from build123d import *

# Parameters (mm, degrees)
CYLINDER005_R     = 2
CYLINDER005_DEPTH = 6
CYLINDER004_R     = 52
CYLINDER004_DEPTH = 67
CYLINDER003_R     = 8
CYLINDER003_DEPTH = 5


with BuildPart() as screw_cut:
    # Cylinder005 → Cylinder005 (new body)
    with BuildSketch(Plane(origin=(0, 56, -0.5), x_dir=(1, 0, 0), z_dir=(0, 0, 1))):
        Circle(CYLINDER005_R)
    extrude(amount=CYLINDER005_DEPTH)


with BuildPart() as cylinder:
    # Cylinder004 → Cylinder004 (new body)
    with BuildSketch(Plane.XY):
        Circle(CYLINDER004_R)
    extrude(amount=CYLINDER004_DEPTH)


with BuildPart() as hinge_final:
    # Cylinder003 → Cylinder003 (new body)
    with BuildSketch(Plane(origin=(0, 52, 0), x_dir=(1, 0, 0), z_dir=(0, 0, 1))):
        Circle(CYLINDER003_R)
    extrude(amount=CYLINDER003_DEPTH)

    # Cut002: cut Cylinder
    add(cylinder.part, mode=Mode.SUBTRACT)

    # Cut003: cut Screw Cut
    add(screw_cut.part, mode=Mode.SUBTRACT)


with BuildPart() as part_mirroring:
    # Part__Mirroring: instance of Hinge Final
    add(hinge_final.part.mirror(Plane(origin=(0.001259, 0, 2.5), x_dir=(1, 0, 0), z_dir=(0, 1, 0))))


solid = part_mirroring.part
Source: CAD feature listing. Evaluate the final solid. Frame: model axes, mm. Round coordinates to 2 decimals unless told otherwise and drop trailing zeros. Loops run counter-clockwise (first coordinate to the right, second up) from the corner with the lowest first, then second, coordinate; pieces in that order, holes last. Notation, with made-up numbers: (14.25, 30) - (36.25, 30) arc R6 ccw to (36.25, 40) - close; hole circle Ø5 at (39.5, -13.75). An arc over 180 degrees is marked (long way). Write item = value, one per line. Start each with the question number.
Item 1: Mould query, pull axis X, two halves, no side actions, for faces 1 (the face through (0, -60, 2)), 2 (the face through (-0.1, -53.8, 0)), 3 (the face through (0, -52, 2)). Classes: released by +X, released by -X, zero draft, split by the parting line, or undercut.
Item 2: Material intervals for line 1 (X direction, y = -57.5, z = 4); line 2 (Y direction, x = 0.75, z = 4.2); line 3 (Y direction, x = 3.5, z = 1.6), sorted ascending.
Item 3: First-contact query: pin 1 Ø1.5 at (y, z) = (-56, 1.5) entering from +X; pin 2 Ø3.5 at (x, y) = (0, -56) entering from -Z. Flat tips, straight axial feed; report the tip coordinate or a pass-through.
Item 4: Section query B-B on y = -56. Output: boundary loops of the cut face in (x, z), plus the area to 3 significant figures.
Item 5: Section query D-D on x = 5. Output: boundary loops of the cut face in (y, z) (3 decimals).
Item 6: Section query A-A on x = 0. Output: boundary loops of the cut face in (y, z).
Item 7: Section query C-C on z = 1.05. Output: boundary loops of the cut face in (x, y).
Results list:
q1.face_1 = split by the parting line
q1.face_2 = zero draft
q1.face_3 = undercut
q2.line_1 = -5.81 to -1.32, 1.32 to 5.81
q2.line_2 = -59.96 to -57.85, -54.15 to -51.99
q2.line_3 = -59.19 to -51.88
q3.pin_1 = 7.31
q3.pin_2 = through
q4.outline = (-6.93, 0) - (-2, 0) - (-2, 5) - (-6.93, 5) - close; (2, 0) - (6.93, 0) - (6.93, 5) - (2, 5) - close
q4.area = 49.3 mm²
q5.outline = (-58.245, 0) - (-51.759, 0) - (-51.759, 5) - (-58.245, 5) - close
q6.outline = (-60, 0) - (-58, 0) - (-58, 5) - (-60, 5) - close; (-54, 0) - (-52, 0) - (-52, 5) - (-54, 5) - close
q7.outline = (-7.98, -51.38) arc R8 ccw (long way) to (7.98, -51.38) arc R52 cw to start; hole circle Ø4 at (0, -56)
